Geometry check sheet. Reference: the model listing, model coordinates, mm. Face numbers are marked on the shaded views. A direction names the side the tool comes from. Round coordinates to 2 decimals unless told otherwise and drop trailing zeros. Order: outer loops, then holes, each group sorted by start corner. A loop starts at its lowest first (then second) coordinate and runs counter-clockwise, first axis right, second up. Notation, with made-up numbers: (50, 78.5) -> (60, 78.5) arc R29 ccw to (60, 111.5) -> close; hole circle Ø6 at (-5, -34.75). An arc over 180 degrees is marked (long way). Answer as a JSON object with one key per item and string values. Group by question number.
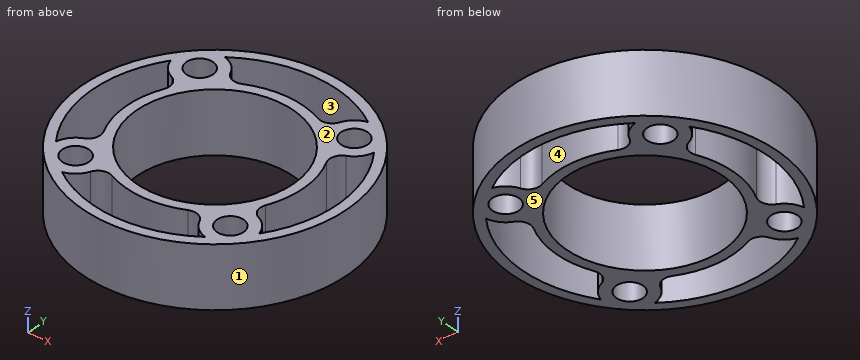
from build123d import *

# Parameters (mm, degrees)
F0_R            = 21.43125
F0_R_2          = 2.15265
F0_R_3          = 12.7
F1_DEPTH        = 9.9568
F3_DEPTH        = 9.9568
F3_COPIES_COUNT = 4
F4_R            = 1.984375


# Not quite as in the source:
# - a pattern or mirror of a feature is missing from the dataset's text; its kind, count and spacing are read off the source's solid


with BuildPart() as f1:
    # F0 (on Top) → F1 (new body)
    with BuildSketch(Plane.XY):
        Circle(F0_R)
        with Locations((-12.3478521665, -12.3478521665)):
            Circle(F0_R_2, mode=Mode.SUBTRACT)
        with Locations((12.3478521665, -12.3478521665)):
            Circle(F0_R_2, mode=Mode.SUBTRACT)
        with Locations((-12.3478521665, 12.3478521665)):
            Circle(F0_R_2, mode=Mode.SUBTRACT)
        Circle(F0_R_3, mode=Mode.SUBTRACT)
        with Locations((12.3478521665, 12.3478521665)):
            Circle(F0_R_2, mode=Mode.SUBTRACT)
    extrude(amount=F1_DEPTH)

    # F2 (on face) → F3 (cut, through all)
    with BuildSketch(Plane.XY.offset(9.9568)):
        with BuildLine():
            ThreePointArc((8.4692641257, 11.5067033254), (8.9929440308, 14.4681276118), (11.4430257563, 16.212081162))
            ThreePointArc((11.4430257563, 16.212081162), (0, 19.84375), (-11.4430257563, 16.212081162))
            ThreePointArc((-11.4430257563, 16.212081162), (-8.9929440308, 14.4681276118), (-8.4692641257, 11.5067033254))
            ThreePointArc((-8.4692641257, 11.5067033254), (0, 14.2875), (8.4692641257, 11.5067033254))
        make_face()
    f3 = extrude(amount=-F3_DEPTH, mode=Mode.SUBTRACT)

    # F3_copies: F3 ×4 about axis
    f3_copies_axis = Axis((0, 0, 0), (0, 0, 1))
    for i in range(1, F3_COPIES_COUNT):
        add(f3.rotate(f3_copies_axis, i * 360 / F3_COPIES_COUNT), mode=Mode.SUBTRACT)

    # F4
    f4_edges = [f1.edges().sort_by_distance(p)[0] for p in [
        (8.469264, 11.506703, 4.9784),
        (-8.469264, 11.506703, 4.9784),
        (8.469264, -11.506703, 4.9784),
        (-8.469264, -11.506703, 4.9784),
        (11.506703, 8.469264, 4.9784),
        (11.506703, -8.469264, 4.9784),
        (-11.506703, -8.469264, 4.9784),
        (-11.506703, 8.469264, 4.9784),
    ]]
    fillet(f4_edges, radius=F4_R)


solid = f1.part
Item 1: Mould release check, pull along Y, two halves, no side actions. Record for the marked faces 1, 2 and 3: pulls with the +Y half, pulls with the -Y half, needs draft (parallel to the pull), parting line crosses it, or undercut.
Item 2: Set-up check for the marked faces 4 and 5: record each of +Z, -Z, +X, -X, +Y, -Y from which the full face is reachable in a straight line by a thin tool's end or side.
Item 3: Sectioned sample at C-C, the plane x = -18. Enter the section's corners in (y, z), then the cut area to 3 significant figures.
Item 4: Thickness scan on L1, parallel to Y at x = -6.5, z = 0.5; L2, parallel to Y at x = 5, z = 8.5; L3, parallel to X at y = -9, z = 6.75. Record the ranges inside material, lowest first.
Item 5: Sectioned sample at A-A, the plane y = 0. Enter the section's corners in (x, z), then the cut area to 3 significant figures.
Item 6: Sectioned sample at D-D, the plane z = 5. Count the separate pieces of the cut face and the enclosed holes in it, then the cut area to 3 significant figures.
Item 7: Depth check by flat-ended pin: pin 1 Ø5 at (x, z) = (7.5, 7.5) entering from -Y; pin 2 Ø2 at (y, z) = (11.5, 6) entering from -X; pin 3 Ø5 at (x, z) = (-8, 2.5) entering from -Y; pin 4 Ø2.5 at (x, y) = (-12.35, 12.35) entering from +Z. Enter the tip coordinate at first touch or a pass-through.
Result:
{
 "1": {"face 1": "parting line crosses it", "face 2": "needs draft", "face 3": "undercut"},
 "2": {"face 4": "+Z, -Z", "face 5": "-Z, +X, -X, +Y, -Y"},
 "3": {"outline": "(-11.63, 0) -> (-8.35, 0) -> (-8.35, 9.96) -> (-11.63, 9.96) -> close; (8.35, 0) -> (11.63, 0) -> (11.63, 9.96) -> (8.35, 9.96) -> close", "area": "65.3 mm2"},
 "4": {"L1": "y = -20.42 to -18.75, -12.79 to -10.91, 10.91 to 12.79, 18.75 to 20.42", "L2": "y = -20.84 to -19.2, -13.38 to -11.67, 11.67 to 13.38, 19.2 to 20.84", "L3": "x = -19.45 to -17.69, -14.48 to -8.96, 8.96 to 14.48, 17.69 to 19.45"},
 "5": {"outline": "(-21.43, 0) -> (-19.84, 0) -> (-19.84, 9.96) -> (-21.43, 9.96) -> close; (-14.29, 0) -> (-12.7, 0) -> (-12.7, 9.96) -> (-14.29, 9.96) -> close; (12.7, 0) -> (14.29, 0) -> (14.29, 9.96) -> (12.7, 9.96) -> close; (19.84, 0) -> (21.43, 0) -> (21.43, 9.96) -> (19.84, 9.96) -> close", "area": "63.2 mm2"},
 "6": {"separate pieces": "1", "enclosed holes": "9", "area": "452 mm2"},
 "7": {"pin 1": "stops at y = -20.84", "pin 2": "stops at x = -18.68", "pin 3": "stops at y = -20.71", "pin 4": "passes through"}
}
